from build123d import *

# Parameters (mm, degrees)
ESBO_O2_R                = 2.5
RESSALTO_EXTRUS_O2_DEPTH = 5
RESSALTO_EXTRUS_O3_DEPTH = 173.55
RESSALTO_EXTRUS_O4_DEPTH = 276.45


with BuildPart() as part:
    # Esbo_o2 → Ressalto-extrus_o2 (new body)
    # profile 1 of 2: a face of its own
    with BuildSketch(Plane(origin=(0, 0, 0), x_dir=(0, 0, -1), z_dir=(1, 0, 0))):
        with BuildLine():
            Line((27.044906217, -7.661000215), (16.526427317, 22.814878798))
            Line((16.526427317, 22.814878798), (-11.047978387, 3.985533348))
            Line((-11.047978387, 3.985533348), (-37.30105887, -13.941537387))
            ThreePointArc((-37.30105887, -13.941537387), (-45.271053286, -17.947334992), (-36.526951093, -16.184410638))
            Line((-36.526951093, -16.184410638), (24.022721227, -12.209541831))
            ThreePointArc((24.022721227, -12.209541831), (32.261148153, -14.405110119), (27.044906217, -7.661000215))
        make_face()
        with Locations((-41.017286054, -16.479185022)):
            Circle(ESBO_O2_R, mode=Mode.SUBTRACT)
        with Locations((28.513056188, -11.914767447)):
            Circle(ESBO_O2_R, mode=Mode.SUBTRACT)
    # profile 2 of 2: a face of its own
    with BuildSketch(Plane(origin=(0, 0, 0), x_dir=(0, 0, -1), z_dir=(1, 0, 0))):
        Polygon((-11.047978387, 3.985533348), (16.526427317, 22.814878798), (92.896691956, 113.919418087), (95.787558299, 117.368025311), (92.071137464, 114.830661289), (1.415245238, 52.935894913), (-2.301175596, 50.398530891), (-3.134557188, 45.976373598), align=None)
    extrude(amount=RESSALTO_EXTRUS_O2_DEPTH)



with BuildPart() as body_2:
    # Esbo_o3 → Ressalto-extrus_o3 (new body)
    with BuildSketch(Plane(origin=(5, 0, 0), x_dir=(0, 0, -1), z_dir=(1, 0, 0))):
        with BuildLine():
            Line((-2.301175596, 50.398530891), (-234.560960335, -108.175443308))
            Line((-234.560960335, -108.175443308), (-266.813676347, -60.935605143))
            Line((-266.813676347, -60.935605143), (-213.363286032, -24.442671921))
            ThreePointArc((-213.363286032, -24.442671921), (-114.312493315, 70.398103063), (10.084451972, 128.114930253))
            Line((10.084451972, 128.114930253), (63.534842287, 164.607863476))
            Line((63.534842287, 164.607863476), (95.787558299, 117.368025311))
            Line((95.787558299, 117.368025311), (-2.301175596, 50.398530891))
        make_face()
    extrude(amount=RESSALTO_EXTRUS_O3_DEPTH)


with BuildPart() as part_1:
    add(part.part)

    add(body_2.part)  # Ressalto-extrus_o4 merges body 2
    # Esbo_o4 → Ressalto-extrus_o4 (add)
    with BuildSketch(Plane.ZY.offset(-5)):
        with BuildLine():
            Line((234.560960335, -108.175443308), (-95.787558299, 117.368025311))
            Line((-95.787558299, 117.368025311), (-63.534842287, 164.607863476))
            Line((-63.534842287, 164.607863476), (-10.084451972, 128.114930253))
            ThreePointArc((-10.084451972, 128.114930253), (114.312493315, 70.398103063), (213.363286032, -24.442671921))
            Line((213.363286032, -24.442671921), (266.813676347, -60.935605143))
            Line((266.813676347, -60.935605143), (234.560960335, -108.175443308))
        make_face()
    extrude(amount=RESSALTO_EXTRUS_O4_DEPTH)


solid = part_1.part
Work out the finished part from the listing and answer in its coordinate system (mm). A direction names the side the tool comes from. Round coordinates to 2 decimals unless told otherwise and drop trailing zeros. Order: outer loops, then holes, each group sorted by start corner. A loop starts at its lowest first (then second) coordinate and runs counter-clockwise, first axis right, second up. Notation, with made-up numbers: M 55.5,-8 L 104.5,-8 A25 cw 104.5,10 Z; hole C -35.5,65.25 d4. An arc over 180 degrees is marked long. Put each result on its own line as item: value. Start each with the question number.
Q1. Section B-B, the plane x = 102 is taken. Write down the section's boundary in (y, z), and give its area (3 significant figures).
Q2. Straight lines are drawn through the part: L1, parallel to Y at x = 30, z = -2; L2, parallel to Y at x = -246, z = 236; L3, parallel to X at y = -7.5, z = -2. For each, find the intervals that lie inside material, in ascending order. Write a range as [from, to].
Q3. Section D-D, the plane z = 81 is taken. Write down the section's boundary in (x, y), and give its area (3 significant figures).
Q4. Section A-A, the plane z = 25 is taken. Write down the section's boundary in (x, y), and give its area (3 significant figures).
Q5. For a pull along Y with two mould halves and no side action, classify faces 4 (the flat face through (-271.45, 39, 86)), 5 (the flat face through (2.46, 7.36, -21.86)), 6 (the flat face through (-43.3, 140.657, -79.887)), 7 (the flat face through (2.46, -4.85, 23.99)) as pulls with the +Y half, pulls with the -Y half, needs draft (parallel to the pull), parting line crosses it, or undercut.
Q6. A tool of negligible diameter and unlimited length cuts with its end or side. For faces 1 (the flat face through (5, 33, -20)), 2 (the flat face through (178.55, 39, 85)), 3 (the flat face through (0, 33, -20)), from which of +Z, -Z, +X, -X, +Y, -Y can it reach the whole face along a straight path? Write none if from no direction.
Q7. Flat-ended cylindrical pins translate along their axes: pin 1 (8 mm diameter, centred on x = -141, z = 117, fed in from -Y); pin 2 (12 mm diameter, centred on x = 117.5, z = 194.5, fed in from -Y); pin 3 (8 mm diameter, centred on x = -29, y = -40.5, fed in from -Z); pin 4 (4 mm diameter, centred on y = -16.48, z = 41.02, fed in from -X). Find the tip coordinate at first contact, or state that the pin passes through.
Q8. Section C-C, the plane y = 58.5 is taken. Write down the section's boundary in (x, z).
Findings below:
1. outline: M -108.18,234.56 L 117.37,-95.79 L 164.61,-63.53 L 128.11,-10.08 A418.36 ccw -24.44,213.36 L -60.94,266.81 Z
1. area: 27,000 mm^2
2. L1: y = [53.34, 125.79]
2. L2: y = [-106.07, -39.9]
2. L3: x = [0, 5]
3. outline: M -271.45,-3.33 L 178.55,-3.33 L 178.55,90.93 L -271.45,90.93 Z
3. area: 42,400 mm^2
4. outline: M -271.45,34.9 L 178.55,34.9 L 178.55,116.73 L -271.45,116.73 Z; M 0,-15.43 L 5,-15.43 L 5,-5.54 L 0,-5.54 Z
4. area: 36,900 mm^2
5. face 4: needs draft
5. face 5: undercut
5. face 6: pulls with the +Y half
5. face 7: undercut
6. face 1: -Z, +X, -Y
6. face 2: +Z, -Z, +X, +Y, -Y
6. face 3: -Z, -X, -Y
7. pin 1: stops at y = -30.64
7. pin 2: stops at y = -84.92
7. pin 3: stops at z = 129.58
7. pin 4: passes through
8. outline: M -271.45,-9.56 L 0,-9.56 L 0,-46.44 L 5,-46.44 L 5,-9.56 L 178.55,-9.56 L 178.55,130.86 L -271.45,130.86 Z
